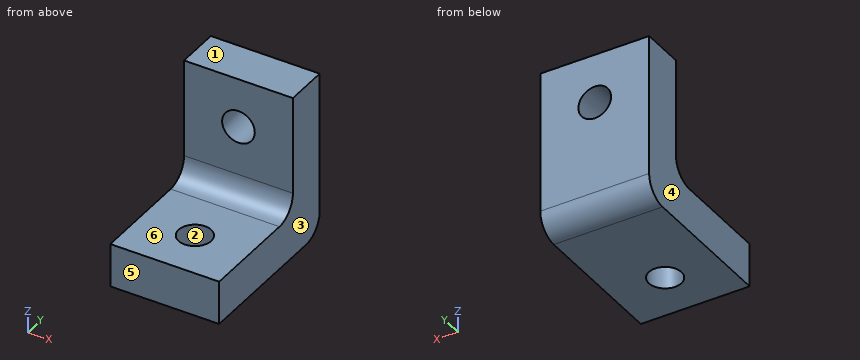
```python
from build123d import *

# Parameters (mm, degrees)
BOSS_EXTRUDE1_DEPTH = 10
SKETCH2_R           = 1.5
CUT_EXTRUDE2_DEPTH  = 22.118712082
SKETCH3_R           = 1.5
CUT_EXTRUDE3_DEPTH  = 22.118712082
FILLET1_R           = 2


with BuildPart() as part:
    # Sketch1 → Boss-Extrude1 (new body)
    with BuildSketch(Plane.YZ):
        with BuildLine():
            Line((0, 0), (0, 15))
            Line((0, 15), (-4, 15))
            Line((-4, 15), (-4, 6))
            ThreePointArc((-4, 6), (-4.585786438, 4.585786438), (-6, 4))
            Line((-6, 4), (-15, 4))
            Line((-15, 4), (-15, 0))
            Line((-15, 0), (0, 0))
        make_face()
    extrude(amount=BOSS_EXTRUDE1_DEPTH)

    # Sketch2 → Cut-Extrude2 (cut, through all)
    with BuildSketch(Plane.XZ.offset(4)):
        with Locations(Location((5, 10.5, 0), (0, 0, 270))):
            Circle(SKETCH2_R)
    extrude(amount=-CUT_EXTRUDE2_DEPTH, mode=Mode.SUBTRACT)

    # Sketch3 → Cut-Extrude3 (cut, through all)
    with BuildSketch(Plane.XY.offset(4)):
        with Locations((5, -10.5)):
            Circle(SKETCH3_R)
    extrude(amount=-CUT_EXTRUDE3_DEPTH, mode=Mode.SUBTRACT)

    # Fillet1
    fillet1_edges = [part.edges().sort_by_distance(p)[0] for p in [
        (5, 0, 0),
    ]]
    fillet(fillet1_edges, radius=FILLET1_R)


solid = part.part
```
Design review of the part built by this model. Coordinates are the model's own, in mm. Face numbers are marked on the shaded views. A direction names the side the tool comes from. Give positions to 0.01 mm unless a question says otherwise; leave off trailing zeros. Order: outer loops, then holes, each group sorted by start corner. A loop starts at its lowest first (then second) coordinate and runs counter-clockwise, first axis right, second up. Notation, with made-up numbers: (-16, -10.75) -> (37, -10.75) arc R26 cw to (37, 25.25) -> close; hole circle Ø8 at (52.5, 48.5). An arc over 180 degrees is marked (long way). Write item = value, one per line. Start each with the question number.
(1) We need section D-D on x = 2.25. Write out the cut boundary in (y, z), plus the area to 3 significant figures.
(2) For the marked faces 5 and 6, list the 3-axis set-ups (+Z, -Z, +X, -X, +Y, -Y) from which the entire face can be reached by the end or side of a thin tool; tool diameter is ignored.
(3) To check wall thickness, follow line 1 along Y through (x, z) = (5, 3.1); line 2 along X through (y, z) = (-2.55, 10.5); line 3 along Y through (x, z) = (2, 14). State the ranges of each line that lie inside material, in increasing order.
(4) We need section C-C on y = -10.5. Write out the cut boundary in (x, z).
(5) We need section A-A on z = 10.5. Write out the cut boundary in (x, y), plus the area to 3 significant figures.
(6) For pin 1 (6 mm diameter, centred on y = -5.5, z = 6.5, fed in from -X); pin 2 (1.8 mm diameter, centred on x = 5, y = -10.5, fed in from +Z); pin 3 (1.5 mm diameter, centred on x = 1.5, y = -6.5, fed in from +Z); pin 4 (4.5 mm diameter, centred on x = 2.5, z = 10.5, fed in from -Y), all flat-tipped, find the tip position at first contact; note any pin that passes through.
(7) Mouldability with a two-part tool opening along X and no side actions: class the marked faces 1, 2, 3 and 4 as +X half, -X half, draft (parallel to the pull), parting line (faces both ways), or undercut.
(8) We need section B-B on x = 5. Write out the cut boundary in (y, z), plus the area to 3 significant figures.
Numbers:
q1.outline = (-15, 0) -> (-2, 0) arc R2 ccw to (0, 2) -> (0, 15) -> (-4, 15) -> (-4, 6) arc R2 cw to (-6, 4) -> (-15, 4) -> close
q1.area = 104 mm^2
q2.face_5 = +Z, -Z, +X, -X, -Y
q2.face_6 = +Z, +X, -X, -Y
q3.line_1 = -15 to -12, -9 to 0
q3.line_2 = 0 to 3.5, 6.5 to 10
q3.line_3 = -4 to 0
q4.outline = (0, 0) -> (3.5, 0) -> (3.5, 4) -> (0, 4) -> close; (6.5, 0) -> (10, 0) -> (10, 4) -> (6.5, 4) -> close
q5.outline = (0, -4) -> (3.5, -4) -> (3.5, 0) -> (0, 0) -> close; (6.5, -4) -> (10, -4) -> (10, 0) -> (6.5, 0) -> close
q5.area = 28.0 mm^2
q6.pin_1 = 0
q6.pin_2 = through
q6.pin_3 = 4.02
q6.pin_4 = -4
q7.face_1 = draft
q7.face_2 = undercut
q7.face_3 = +X half
q7.face_4 = -X half
q8.outline = (-15, 0) -> (-12, 0) -> (-12, 4) -> (-15, 4) -> close; (-9, 0) -> (-2, 0) arc R2 ccw to (0, 2) -> (0, 9) -> (-4, 9) -> (-4, 6) arc R2 cw to (-6, 4) -> (-9, 4) -> close; (-4, 12) -> (0, 12) -> (0, 15) -> (-4, 15) -> close
q8.area = 80.0 mm^2
